The model under review builds one solid part; all positions refer to its coordinate system, in mm. A direction names the side the tool comes from. Round coordinates to 2 decimals unless told otherwise and drop trailing zeros. Order: outer loops, then holes, each group sorted by start corner. A loop starts at its lowest first (then second) coordinate and runs counter-clockwise, first axis right, second up. Notation, with made-up numbers: M -34.75,73 L -29.75,73 A30 cw -29.75,100 Z; hole C -15,78.5 d1. An arc over 180 degrees is marked long. Answer as CSV lines item,"result". Start each with the question number.
from build123d import *

# Parameters (mm, degrees)
SKETCH1_W               = 14
SKETCH1_H               = 3.5
BOSS_EXTRUDE1_DEPTH     = 1.9
CUT_EXTRUDE1_DEPTH      = 8.461400673
CUT_EXTRUDE1_DEPTH_BACK = 8.461400673
SKETCH4_W               = 0.07
SKETCH4_H               = 0.024
BOSS_EXTRUDE3_DEPTH     = 10
SWEEP1_START            = -1.75
SWEEP1_DEPTH            = 3.5


# Read off the part's stored shape, not the designer's step: Sweep1
with BuildPart() as part:
    # Sketch1 → Boss-Extrude1 (new body)
    with BuildSketch(Plane(origin=(0, 0, 0), x_dir=(1, 0, 0), z_dir=(0, 1, 0))):
        Rectangle(SKETCH1_W, SKETCH1_H)
    extrude(amount=BOSS_EXTRUDE1_DEPTH)

    # Sketch3 → Cut-Extrude1 (cut, two sides: drawn at the far end of the back side and taken through both)
    with BuildSketch(Plane.XY.offset(-CUT_EXTRUDE1_DEPTH_BACK)):
        with BuildLine():
            Line((7, 0.6), (7, 1.9))
            Line((7, 1.9), (2, 1.9))
            ThreePointArc((2, 1.9), (3.291559135, 1.734842828), (4.5, 1.25))
            ThreePointArc((4.5, 1.25), (5.708440865, 0.765157172), (7, 0.6))
        make_face()
    extrude(amount=CUT_EXTRUDE1_DEPTH + CUT_EXTRUDE1_DEPTH_BACK, mode=Mode.SUBTRACT)

    # Sketch4 → Boss-Extrude3 (add)
    with BuildSketch(Plane.ZY.offset(7)):
        with Locations((0, 0.5)):
            Rectangle(SKETCH4_W, SKETCH4_H)
    extrude(amount=BOSS_EXTRUDE3_DEPTH)

    # Sweep1 outline → Sweep1 (add)
    with BuildSketch(Plane.XY.offset(SWEEP1_START)):
        with BuildLine():
            Line((10.549140882, -6.409601789), (7.549140882, -6.409601789))
            Line((7.549140882, -6.409601789), (7.549140882, -6.909601789))
            Line((7.549140882, -6.909601789), (10.549140882, -6.909601789))
            ThreePointArc((10.549140882, -6.909601789), (19.285582655, 0.503552751), (13.39347688, 10.330218748))
            ThreePointArc((13.39347688, 10.330218748), (10.067527148, 9.33364199), (9.916983753, 5.864860714))
            ThreePointArc((9.916983753, 5.864860714), (10.053298409, 2.315301648), (7, 0.5))
            Line((7, 0.5), (7, 0))
            ThreePointArc((7, 0), (10.492566046, 2.076462911), (10.336640265, 6.136684944))
            ThreePointArc((10.336640265, 6.136684944), (10.462056054, 9.026482516), (13.232862483, 9.85671794))
            ThreePointArc((13.232862483, 9.85671794), (18.792251933, 0.584945612), (10.549140882, -6.409601789))
        make_face()
    extrude(amount=SWEEP1_DEPTH)


solid = part.part
Item 1: Consider section D-D (x = -3.5). State the section outline as (y, z) points.
Item 2: Consider section B-B (y = 6.75). State the section outline as (x, z) points, and give its area (3 significant figures).
Item 3: The part is to be moulded in two halves that separate along X. For faces 6 (the cylindrical face through (19.255, 0.332, -0.024)), 7 (the cylindrical face through (10.1, 2.4, 0)), 8 (the flat face through (0, 0, 0)), say which applies: +X half, -X half, draft (parallel to the pull), parting line (faces both ways), or undercut.
Item 4: Consider section A-A (x = 14). State the section outline as (y, z) points, and give its area (3 significant figures).
Item 5: Tool access review of faces 1 (the flat face through (9, -6.91, 0)), 2 (the cylindrical face through (18.817, 0.748, -0.024)), 3 (the flat face through (6.1, 0.5, -1.75)), 4 (the flat face through (-3, 1.9, 0)), 5 (the flat face through (9, -6.41, 0)): name each direction out of +Z, -Z, +X, -X, +Y, -Y from which nothing blocks a thin tool from reaching the whole face with its end or side.
Item 6: Wall thickness on probe 1 along Y at (x, z) = (-3.5, -0.5); probe 2 along X at (y, z) = (2.5, 1.6); probe 3 along X at (y, z) = (8.25, 0.7): over which ranges is each line inside the solid? List them lowest first. Write a range as [from, to].
Item 7: For pin 1 (0.9 mm diameter, centred on x = 8.5, z = 0.5, fed in from +Y); pin 2 (6 mm diameter, centred on x = 6, y = 8, fed in from +Z); pin 3 (1.5 mm diameter, centred on y = 1.5, z = -1, fed in from -X); pin 4 (0.6 mm diameter, centred on y = -6.5, z = 0, fed in from -X), all flat-tipped, find the tip position at first contact; note any pin that passes through.
Item 8: Consider section C-C (z = -1.4). State the section outline as (x, y) points, and give its area (4 significant figures).
Reported:
1,outline,"M 0,-1.75 L 1.9,-1.75 L 1.9,1.75 L 0,1.75 Z"
2,outline,"M 9.53,-1.75 L 10.05,-1.75 L 10.05,1.75 L 9.53,1.75 Z; M 17.38,-1.75 L 17.99,-1.75 L 17.99,1.75 L 17.38,1.75 Z"
2,area,"3.93 mm²"
3,face 6,"+X half"
3,face 7,"undercut"
3,face 8,"draft"
4,outline,"M -6.21,-1.75 L -5.66,-1.75 L -5.66,1.75 L -6.21,1.75 Z; M 9.55,-1.75 L 10.1,-1.75 L 10.1,1.75 L 9.55,1.75 Z"
4,area,"3.82 mm²"
5,face 1,"+Z, -Z, +X, -X, -Y"
5,face 2,"+Z, -Z"
5,face 3,"-Z, +X, -X, +Y, -Y"
5,face 4,"+Z, -Z, -X, +Y"
5,face 5,"+Z, -Z, -X"
6,probe 1,"y = [0, 1.9]"
6,probe 2,"x = [10.15, 10.69], [18.89, 19.39]"
6,probe 3,"x = [9.53, 10.05], [16.03, 16.77]"
7,pin 1,"stops at y = 1.1"
7,pin 2,"passes through"
7,pin 3,"stops at x = -7"
7,pin 4,"stops at x = 7.55"
8,outline,"M -7,0 L 7,0 A3.98 ccw 10.34,6.14 A2.5 cw 13.23,9.86 A8.35 cw 10.55,-6.41 L 7.55,-6.41 L 7.55,-6.91 L 10.55,-6.91 A8.85 ccw 13.39,10.33 A3 ccw 9.92,5.86 A3.48 cw 7,0.5 L 7,0.6 A5.13 cw 4.5,1.25 A5.13 ccw 2,1.9 L -7,1.9 Z"
8,area,"44.35 mm²"
